For this review, take the finished solid that the model builds, in its own axes (mm). Face numbers are marked on the shaded views. A direction names the side the tool comes from. Give positions to 0.01 mm unless a question says otherwise; leave off trailing zeros. Order: outer loops, then holes, each group sorted by start corner. A loop starts at its lowest first (then second) coordinate and runs counter-clockwise, first axis right, second up. Notation, with made-up numbers: (11, 27) - (32, 27) arc R20 cw to (32, 40) - close; hole circle Ø9 at (32.5, 3.25). An arc over 180 degrees is marked (long way). Put each result on its own line as item: value. Start each with the question number.
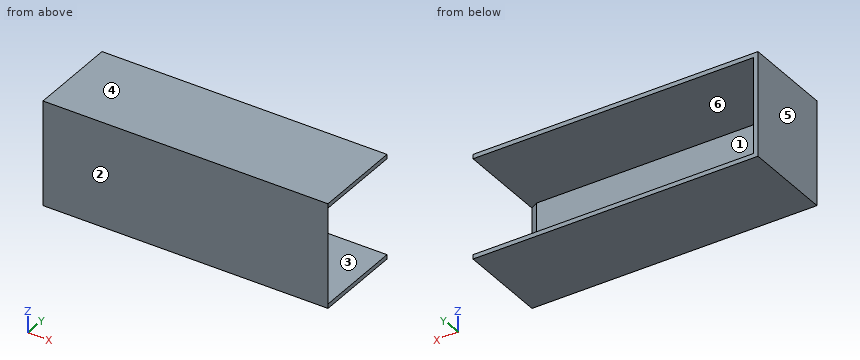
```python
from build123d import *

# Parameters (mm, degrees)
ESQUISSE1_W        = 196
ESQUISSE1_H        = 72
BOSS_EXTRU_1_DEPTH = 3
BOSS_EXTRU_2_DEPTH = 58.8
CHANFREIN1_SIZE    = 2.886751346
CHANFREIN1_SIZE2   = 5


with BuildPart() as part:
    # Esquisse1 → Boss.-Extru.1 (new body)
    with BuildSketch(Plane(origin=(0, 0, 0), x_dir=(1, 0, 0), z_dir=(0, 1, 0))):
        with Locations((60.813158837, -17.029685758)):
            Rectangle(ESQUISSE1_W, ESQUISSE1_H)
    extrude(amount=BOSS_EXTRU_1_DEPTH)

    # Esquisse2 → Boss.-Extru.2 (add)
    with BuildSketch(Plane(origin=(0, 3, 0), x_dir=(1, 0, 0), z_dir=(0, 1, 0))):
        Polygon((-37.186841163, 18.970314242), (158.813158837, 18.970314242), (158.813158837, 15.970314242), (-34.186841163, 15.970314242), (-34.186841163, -50.029685758), (158.813158837, -50.029685758), (158.813158837, -53.029685758), (-37.186841163, -53.029685758), align=None)
    extrude(amount=BOSS_EXTRU_2_DEPTH)

    # Chanfrein1
    chanfrein1_edges = [part.edges().sort_by_distance(p)[0] for p in [
        (158.813158837, 3, 17.029685758),
    ]]
    chanfrein1_side = [part.faces().sort_by_distance(p)[0] for p in [
        (158.813158837, 30.9, -18.021460196),
    ]]
    chamfer(chanfrein1_edges, length=CHANFREIN1_SIZE, length2=CHANFREIN1_SIZE2, reference=chanfrein1_side[0])


solid = part.part
```
1. The part is to be moulded in two halves that separate along Z. For the marked faces 1, 2, 3 and 4, say which applies: released by +Z, released by -Z, zero draft, split by the parting line, or undercut.
2. Wall thickness on line 1 (Z direction, x = 81, y = 39.5); line 2 (X direction, y = 31.5, z = 15.5); line 3 (Y direction, x = 10, z = -7): over which ranges is each line inside the solid? List them lowest first. Write a range as from..to.
3. Clearance check with flat-ended pins moving along their axes: pin 1 (1.5 mm diameter, centred on y = 36.5, z = 32.5, fed in from +X); pin 2 (3 mm diameter, centred on x = -17.5, z = 11, fed in from +Y). State where each tip first meets the part, or that it passes through.
4. Add section B-B, the plane x = -19.5. Give the boundary of the cut face in (y, z).
5. Tool access review of the marked faces 5 and 6: name each direction out of +Z, -Z, +X, -X, +Y, -Y from which nothing blocks a thin tool from reaching the whole face with its end or side.
6. Add section C-C, the plane z = 41. Give the boundary of the cut face in (x, y), then the cut area to 3 significant figures.
7. Add section A-A, the plane y = 11. Give the boundary of the cut face in (x, z).
Found:
1. face 1: undercut
1. face 2: zero draft
1. face 3: undercut
1. face 4: released by +Z
2. line 1: z = -18.97..-15.97, 50.03..53.03
2. line 2: x = -37.19..-34.19
2. line 3: y = 0..3
3. pin 1: stops at x = -34.19
3. pin 2: stops at y = 3
4. outline: (0, -18.97) - (61.8, -18.97) - (61.8, -15.97) - (3, -15.97) - (3, 50.03) - (61.8, 50.03) - (61.8, 53.03) - (0, 53.03) - close
5. face 5: +Z, -Z, -X, +Y, -Y
5. face 6: +X, +Y
6. outline: (-37.19, 0) - (158.81, 0) - (158.81, 0.11) - (153.81, 3) - (-34.19, 3) - (-34.19, 61.8) - (-37.19, 61.8) - close
6. area: 757 mm^2
7. outline: (-37.19, -18.97) - (158.81, -18.97) - (158.81, -15.97) - (-34.19, -15.97) - (-34.19, 50.03) - (158.81, 50.03) - (158.81, 53.03) - (-37.19, 53.03) - close
